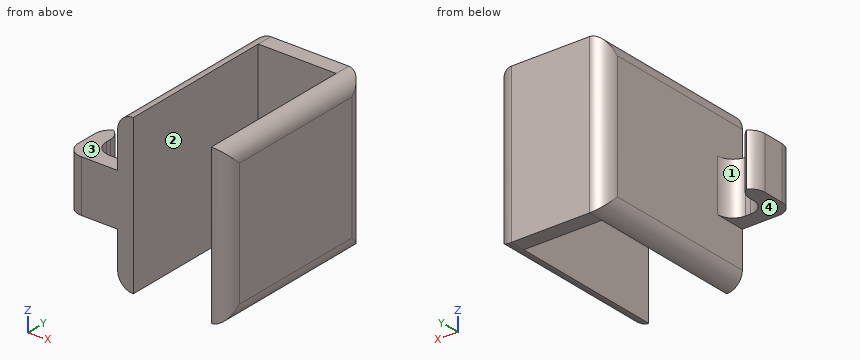
from build123d import *

# Parameters (mm, degrees)
F1_DEPTH    = 30
F2_START    = 10
F2_DEPTH    = 10
F3_T1_DEPTH = 10
F3_T3_DEPTH = 25
F3_T5_DEPTH = 48
F3_T7_DEPTH = 45


# Not quite as in the source:
# - a fillet or chamfer that OpenCascade refuses, or shapes differently, is made with other operations: its cross-section is extruded or revolved along the edge and cut away or added


with BuildPart() as f1:
    # F0 (on Top) → F1 (new body)
    with BuildSketch(Plane.XY):
        Polygon((7.5, 30), (7.5, 0), (10.5, 0), (10.5, 33), (-10.5, 33), (-10.5, 3), (-10.5, 0), (-7.5, 0), (-7.5, 30), align=None)
    extrude(amount=F1_DEPTH)

    # F0 (on Top) → F2 (join)
    with BuildSketch(Plane.XY.offset(F2_START)):
        Polygon((7.5, 30), (7.5, 0), (10.5, 0), (10.5, 33), (-10.5, 33), (-10.5, 3), (-10.5, 0), (-7.5, 0), (-7.5, 30), align=None)
        Polygon((-10.5, 0), (-10.5, 3), (-17.5, 3), (-17.5, 10), (-20.5, 10), (-20.5, 0), align=None)
    extrude(amount=F2_DEPTH)

    # F3: fillet of radius 3 on 12 edges, made by hand

    # F3_s2 → F3_t1 (join)
    with BuildSketch(Plane.XY.offset(10)):
        with BuildLine():
            ThreePointArc((-10.5, 6), (-11.3786796564, 3.8786796564), (-13.5, 3))
            Line((-13.5, 3), (-10.5, 3))
            Line((-10.5, 3), (-10.5, 6))
        make_face()
        with BuildLine():
            ThreePointArc((-17.5, 6), (-16.6213203436, 3.8786796564), (-14.5, 3))
            Line((-14.5, 3), (-17.5, 3))
            Line((-17.5, 3), (-17.5, 6))
        make_face()
    extrude(amount=F3_T1_DEPTH)

    # F3_s4 → F3_t3 (cut)
    with BuildSketch(Plane.XY.offset(2.5)):
        with BuildLine():
            ThreePointArc((-20.5, 10), (-18.3786796564, 9.1213203436), (-17.5, 7))
            Line((-17.5, 7), (-17.5, 10))
            Line((-17.5, 10), (-20.5, 10))
        make_face()
        with BuildLine():
            ThreePointArc((-20.5, 3), (-19.6213203436, 0.8786796564), (-17.5, 0))
            Line((-17.5, 0), (-20.5, 0))
            Line((-20.5, 0), (-20.5, 3))
        make_face()
        with BuildLine():
            ThreePointArc((-20.5, 7), (-19.6213203436, 9.1213203436), (-17.5, 10))
            Line((-17.5, 10), (-20.5, 10))
            Line((-20.5, 10), (-20.5, 7))
        make_face()
    extrude(amount=F3_T3_DEPTH, mode=Mode.SUBTRACT)

    # F3_s6 → F3_t5 (cut)
    with BuildSketch(Plane.XZ.offset(-40.5)):
        with BuildLine():
            ThreePointArc((-10.5, 27), (-9.6213203436, 29.1213203436), (-7.5, 30))
            Line((-7.5, 30), (-10.5, 30))
            Line((-10.5, 30), (-10.5, 27))
        make_face()
        with BuildLine():
            ThreePointArc((10.5, 3), (9.6213203436, 0.8786796564), (7.5, 0))
            Line((7.5, 0), (10.5, 0))
            Line((10.5, 0), (10.5, 3))
        make_face()
        with BuildLine():
            ThreePointArc((10.5, 27), (9.6213203436, 29.1213203436), (7.5, 30))
            Line((7.5, 30), (10.5, 30))
            Line((10.5, 30), (10.5, 27))
        make_face()
        with BuildLine():
            ThreePointArc((-10.5, 3), (-9.6213203436, 0.8786796564), (-7.5, 0))
            Line((-7.5, 0), (-10.5, 0))
            Line((-10.5, 0), (-10.5, 3))
        make_face()
    extrude(amount=F3_T5_DEPTH, mode=Mode.SUBTRACT)

    # F3_s8 → F3_t7 (cut)
    with BuildSketch(Plane.XY.offset(-7.5)):
        with BuildLine():
            ThreePointArc((7.5, 0), (9.6213203436, 0.8786796564), (10.5, 3))
            Line((10.5, 3), (10.5, 0))
            Line((10.5, 0), (7.5, 0))
        make_face()
        with BuildLine():
            ThreePointArc((10.5, 30), (9.6213203436, 32.1213203436), (7.5, 33))
            Line((7.5, 33), (10.5, 33))
            Line((10.5, 33), (10.5, 30))
        make_face()
        with BuildLine():
            ThreePointArc((-7.5, 33), (-9.6213203436, 32.1213203436), (-10.5, 30))
            Line((-10.5, 30), (-10.5, 33))
            Line((-10.5, 33), (-7.5, 33))
        make_face()
    extrude(amount=F3_T7_DEPTH, mode=Mode.SUBTRACT)


solid = f1.part
Build history of the part. All positions in model axes, mm. Face numbers are marked on the shaded views. A direction names the side the tool comes from. Coordinates: 2 decimals unless noted, no trailing zeros. Order: outer loops, then holes, each group sorted by start corner. A loop starts at its lowest first (then second) coordinate and runs counter-clockwise, first axis right, second up. Notation, with made-up numbers: (37.25, 54) - (45.25, 54) arc R25 ccw to (45.25, 73) - close; hole circle Ø8 at (34, -35.5). An arc over 180 degrees is marked (long way). Write each question's results on one line, items separated by ' | '. Start each with the question number.
Item 1: Tool access for the marked faces 1, 2, 3 and 4: list every direction of +Z, -Z, +X, -X, +Y, -Y with a clear straight run to the whole face (end or side of a thin tool).
Item 2: Band-saw the part on D-D on z = 5.25. Write the cut outline in (x, y), and give its area (3 significant figures).
Item 3: Band-saw the part on B-B on z = 18.5. Write the cut outline in (x, y), and give its area (3 significant figures).
Item 4: Wall check: probe 1 along X at (y, z) = (26, 14); probe 2 along Y at (x, z) = (2, 27.5); probe 3 along Y at (x, z) = (-13.5, 12.25). Give the ranges that are in metal, low to high. Write a range as [from, to].
Item 5: Band-saw the part on C-C on x = 1. Write the cut outline in (y, z).
Item 6: Band-saw the part on A-A on y = 16. Write the cut outline in (x, z), and give its area (3 significant figures).
Item 7: Flat gauge pins, fed straight in: pin 1 (2 mm diameter, centred on x = -11, y = 15.5, fed in from +Z); pin 2 (7.5 mm diameter, centred on x = -13.5, y = 6.5, fed in from -Z); pin 3 (1 mm diameter, centred on x = -9.5, z = 4.5, fed in from +Y); pin 4 (1.5 mm diameter, centred on x = -16, z = 21.5, fed in from -Y) (1 decimal). Where does each tip first touch, or does it go through?
Numbers:
1) face 1: +Z, -Z, +Y | face 2: +Z, -Z, -Y | face 3: +Z, -X, +Y, -Y | face 4: -Z, -X, +Y, -Y
2) outline: (-10.5, 0) - (-7.5, 0) - (-7.5, 30) - (7.5, 30) - (7.5, 0) arc R3 ccw to (10.5, 3) - (10.5, 30) arc R3 ccw to (7.5, 33) - (-7.5, 33) arc R3 ccw to (-10.5, 30) - close | area: 237 mm^2
3) outline: (-20.5, 3) arc R3 ccw to (-17.5, 0) - (-7.5, 0) - (-7.5, 30) - (7.5, 30) - (7.5, 0) arc R3 ccw to (10.5, 3) - (10.5, 30) arc R3 ccw to (7.5, 33) - (-7.5, 33) arc R3 ccw to (-10.5, 30) - (-10.5, 6) arc R3 cw to (-13.5, 3) - (-14.5, 3) arc R3 cw to (-17.5, 6) - (-17.5, 7) arc R3 ccw to (-19, 9.6) arc R3 ccw to (-20.5, 7) - close | area: 287 mm^2
4) probe 1: [-10.5, -7.5], [7.5, 10.5] | probe 2: [30, 33] | probe 3: [0, 3]
5) outline: (30, 0) - (33, 0) - (33, 30) - (30, 30) - close
6) outline: (-10.5, 3) arc R3 ccw to (-7.5, 0) - (-7.5, 30) arc R3 ccw to (-10.5, 27) - close; (7.5, 0) arc R3 ccw to (10.5, 3) - (10.5, 27) arc R3 ccw to (7.5, 30) - close | area: 172 mm^2
7) pin 1: z = 28.66 | pin 2: z = 1.02 | pin 3: y = 32.6 | pin 4: through
